Here's the drawing with two shaded views (mm, measured from the low corner). I have some questions. A direction names the side the tool comes from. Give positions to 0.01 mm unless a question says otherwise; leave off trailing zeros. One line per item, written item: value.
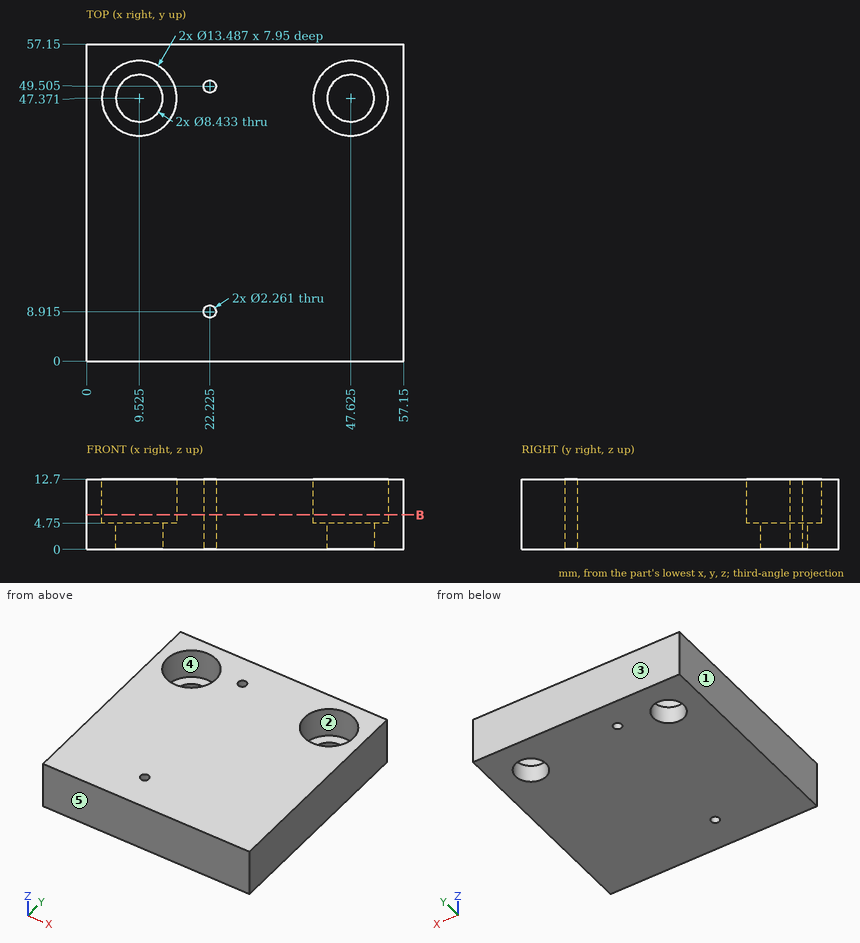
1) We'd pull the mould along X, two halves only. Please class the marked faces 1, 2 and 3: released by +X, released by -X, zero draft, split by the parting line, or undercut.
Answer list:
face 1: released by -X
face 2: undercut
face 3: zero draft
2) I need wall thicknesses on L1, parallel to X at y = 44.5, z = 5; L2, parallel to Y at x = 52.5, z = 6; L3, parallel to Y at x = 8, z = 7.5. Which ranges of each line are inside material? Lowest first, please.
Answer list:
L1: x = 0 to 3.42, 15.63 to 41.52, 53.73 to 57.15
L2: y = 0 to 42.71, 52.03 to 57.15
L3: y = 0 to 40.8, 53.94 to 57.15
3) Will this pin go through, and if not, where does the flat tip stop? pin 1 (11 mm diameter, centred on x = 48, y = 47.5, fed in from +Z).
Answer list:
pin 1: stops at z = 4.75
4) If we section it at B-B (z = 6.25): State how many separate pieces and enclosed holes the cut face has, and give its area (3 significant figures).
Answer list:
separate pieces: 1
enclosed holes: 4
area: 2,970 mm^2
5) For the marked faces 4 and 5, which set-ups out of +Z, -Z, +X, -X, +Y, -Y let a thin tool reach every point of the face, with its end or its side?
Answer list:
face 4: +Z
face 5: +Z, -Z, +X, -X, -Y
